The figure shows three views and two pictorial views of one solid part (mm, origin at its lowest corner). Answer the questions. Round coordinates to 2 decimals unless told otherwise and drop trailing zeros. Write each loop counter-clockwise with the first axis right and the second up, starting at its lowest first coordinate (ties: lowest second). Pieces come first, ordered by that corner, then holes. Notation, with made-up numbers: (-10, 41.25) - (28, 41.25) arc R16 ccw to (28, 63.25) - close; hole circle Ø2 at (-33.5, 59.25). An arc over 180 degrees is marked (long way). Answer as CSV lines item,"result". Start each with the question number.
Item 1: A cutting plane is placed at C-C on y = 1.5. Determine the outline of the cut face in (x, z) (1 decimal), and give its area (3 significant figures).
Item 2: Flat-ended cylindrical pins translate along their axes: pin 1 (1 mm diameter, centred on y = 1, z = 23.5, fed in from +X) (1 decimal); pin 2 (1.6 mm diameter, centred on y = 2, z = 32, fed in from -X) (1 decimal). Find the tip coordinate at first contact, or state that the pin passes through.
Item 3: A cutting plane is placed at A-A on z = 45.5. Determine the outline of the cut face in (x, y) (1 decimal), and give its area (3 significant figures).
Item 4: A cutting plane is placed at B-B on x = 45. Determine the outline of the cut face in (y, z) (1 decimal).
Item 5: Straight lines are drawn through the part: line 1 along Z through (x, y) = (45.5, 1.8) (1 decimal); line 2 along X through (y, z) = (1.75, 14) (1 decimal). For each, find the intervals that lie inside material, in ascending order. Write a range as [from, to].
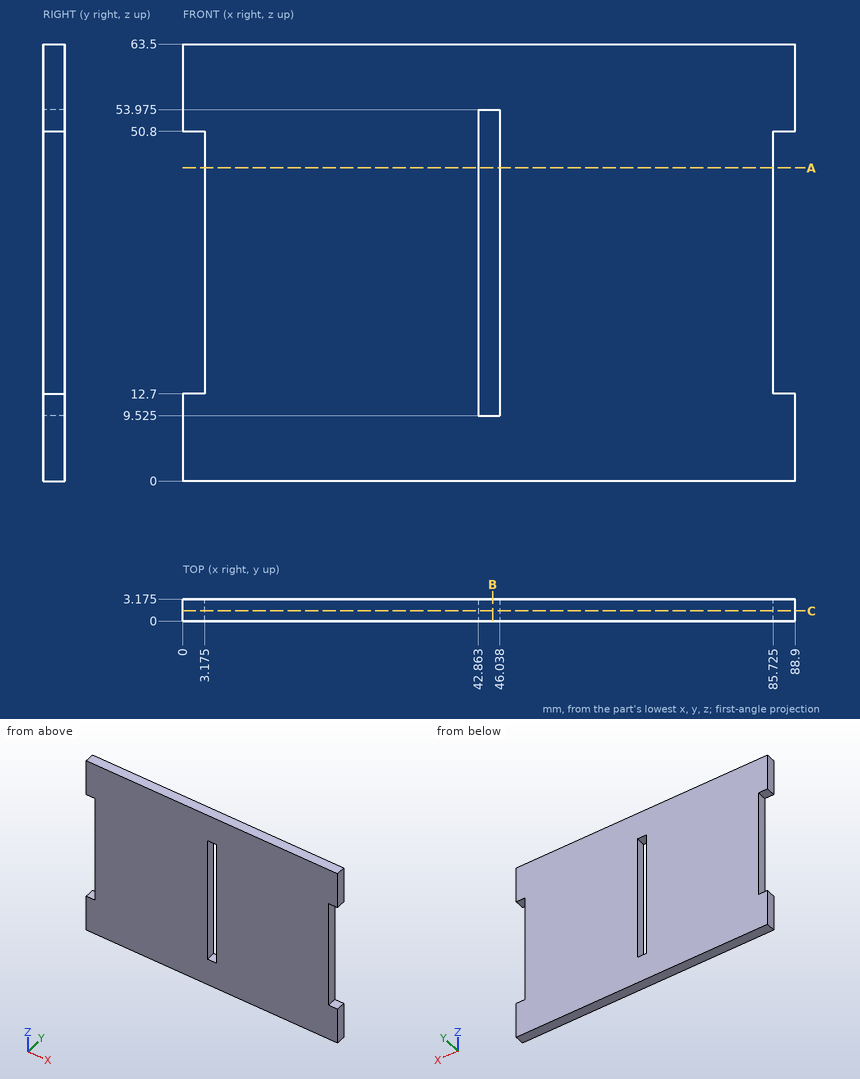
Geometry says:
1,outline,"(0, 0) - (88.9, 0) - (88.9, 12.7) - (85.7, 12.7) - (85.7, 50.8) - (88.9, 50.8) - (88.9, 63.5) - (0, 63.5) - (0, 50.8) - (3.2, 50.8) - (3.2, 12.7) - (0, 12.7) - close; hole (42.9, 9.5) - (46, 9.5) - (46, 54) - (42.9, 54) - close"
1,area,"5,260 mm^2"
2,pin 1,"stops at x = 85.7"
2,pin 2,"stops at x = 3.2"
3,outline,"(3.2, 0) - (42.9, 0) - (42.9, 3.2) - (3.2, 3.2) - close; (46, 0) - (85.7, 0) - (85.7, 3.2) - (46, 3.2) - close"
3,area,"252 mm^2"
4,outline,"(0, 0) - (3.2, 0) - (3.2, 9.5) - (0, 9.5) - close; (0, 54) - (3.2, 54) - (3.2, 63.5) - (0, 63.5) - close"
5,line 1,"z = [0, 9.5], [54, 63.5]"
5,line 2,"x = [3.2, 42.9], [46, 85.7]"
